Model file for the job. Use its own axes, mm. Face numbers are marked on the shaded views. A direction names the side the tool comes from. Give positions to 0.01 mm unless a question says otherwise; leave off trailing zeros. Order: outer loops, then holes, each group sorted by start corner. A loop starts at its lowest first (then second) coordinate and runs counter-clockwise, first axis right, second up. Notation, with made-up numbers: (-21.5, 80.5) -> (32.5, 80.5) arc R4 ccw to (32.5, 87.5) -> close; hole circle Ø10 at (9, 52). An arc over 180 degrees is marked (long way). Answer in a Markdown table with one row per item. Add a question column.
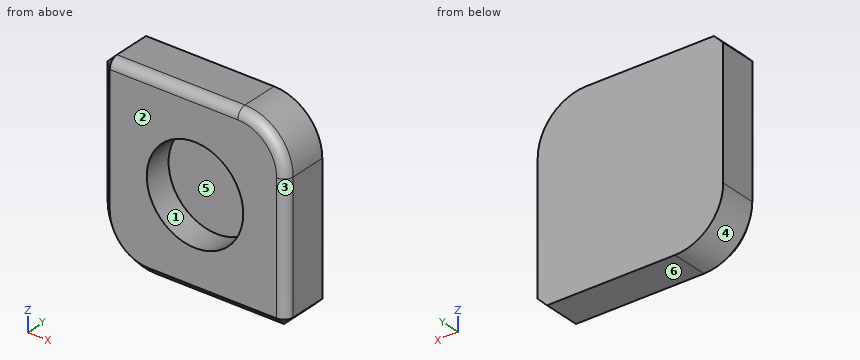
from build123d import *

# Parameters (mm, degrees)
F1_DEPTH = 25
F2_R     = 5
F3_SIZE  = 5
F4_R     = 26.000333
F5_DEPTH = 15


with BuildPart() as f1:
    # F0 (on Front) → F1 (new body)
    with BuildSketch(Plane.XZ):
        with BuildLine():
            Line((30.506836, 50.163411), (-43.493164, 50.163411))
            Line((-43.493164, 50.163411), (-43.493164, -23.836589))
            ThreePointArc((-43.493164, -23.836589), (-35.87794, -42.221365), (-17.493164, -49.836589))
            Line((-17.493164, -49.836589), (56.506836, -49.836589))
            Line((56.506836, -49.836589), (56.506836, 24.163411))
            ThreePointArc((56.506836, 24.163411), (48.891612, 42.548187), (30.506836, 50.163411))
        make_face()
    extrude(amount=F1_DEPTH)

    # F2
    f2_edges = [f1.edges().sort_by_distance(p)[0] for p in [
        (-6.493164, -25, 50.163411),
    ]]
    fillet(f2_edges, radius=F2_R)

    # F3
    f3_edges = [f1.edges().sort_by_distance(p)[0] for p in [
        (-43.493164, -10, 50.163411),
    ]]
    chamfer(f3_edges, length=F3_SIZE)

    # F4 (on face) → F5 (cut)
    with BuildSketch(Plane.XZ.offset(25)):
        with Locations((7.471764, 0)):
            Circle(F4_R)
    extrude(amount=-F5_DEPTH, mode=Mode.SUBTRACT)


solid = f1.part
Item 1: Two-plate mould, pull along X, no slides. Class the marked faces 3, 4, 5 and 6: pulls with the +X half, pulls with the -X half, needs draft (parallel to the pull), parting line crosses it, or undercut.
Item 2: Saw through at C-C on z = 0. List the corners of the cut face in (x, y).
Item 3: Saw through at B-B on x = 8.5. List the corners of the cut face in (y, z), plus the area to 3 significant figures.
Item 4: Which spindle directions (+Z, -Z, +X, -X, +Y, -Y) get a long thin tool onto all of the face, cutting with end or side? Do the marked faces 1 and 2. Say none if no direction does.
Item 5: Wall check: line 1 (Y direction, x = 11.5, z = 22.5); line 2 (Z direction, x = -4, y = -24); line 3 (Z direction, x = -18, y = -2.75). Give the ranges that are in metal, low to high.
Item 6: Saw through at D-D on y = -3.25. List the corners of the cut face in (x, z), plus the area to 3 significant figures.
Item 7: Pin check, flat tips, straight feed: pin 1 Ø4 at (y, z) = (-21, 36) entering from +X; pin 2 Ø4 at (x, z) = (10, -8) entering from -Y. Stop position of each tip, or through.
Item 8: Saw through at A-A on y = -18.25. List the corners of the cut face in (x, z), plus the area to 3 significant figures.
Evaluation:
| question | item | result |
|---|---|---|
| 1 | face 3 | pulls with the +X half |
| 1 | face 4 | pulls with the -X half |
| 1 | face 5 | undercut |
| 1 | face 6 | needs draft |
| 2 | outline | (-43.49, -20) -> (-38.49, -25) -> (-18.53, -25) -> (-18.53, -10) -> (33.47, -10) -> (33.47, -25) -> (51.51, -25) arc R5 ccw to (56.51, -20) -> (56.51, 0) -> (-43.49, 0) -> close |
| 3 | outline | (-25, -44.84) -> (-20, -49.84) -> (0, -49.84) -> (0, 50.16) -> (-20, 50.16) arc R5 ccw to (-25, 45.16) -> (-25, 25.98) -> (-10, 25.98) -> (-10, -25.98) -> (-25, -25.98) -> close |
| 3 | area | 1,700 mm2 |
| 4 | face 1 | -Y |
| 4 | face 2 | +Z, -Z, +X, -X, -Y |
| 5 | line 1 | y = -10 to 0 |
| 5 | line 2 | z = -45.84 to -23.33, 23.33 to 48.16 |
| 5 | line 3 | z = -49.83 to 50.16 |
| 6 | outline | (-43.49, -23.84) arc R26 ccw to (-17.49, -49.84) -> (51.51, -49.84) -> (56.51, -44.84) -> (56.51, 24.16) arc R26 ccw to (30.51, 50.16) -> (-38.49, 50.16) -> (-43.49, 45.16) -> close |
| 6 | area | 9,680 mm2 |
| 7 | pin 1 | stops at x = 54.52 |
| 7 | pin 2 | stops at y = -10 |
| 8 | outline | (-43.49, -23.84) arc R26 ccw to (-17.49, -49.84) -> (51.51, -49.84) -> (56.51, -44.84) -> (56.51, 24.16) arc R26 ccw to (30.51, 50.16) -> (-38.49, 50.16) -> (-43.49, 45.16) -> close; hole circle Ø52 at (7.47, 0) |
| 8 | area | 7,560 mm2 |
